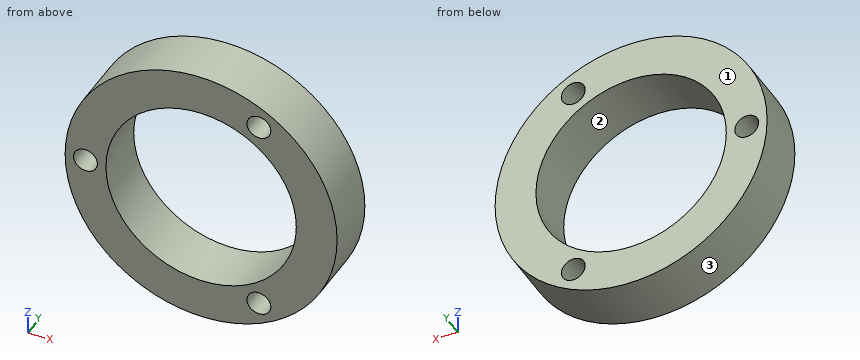
from build123d import *

# Parameters (mm, degrees)
SKETCH1_R           = 20
BOSS_EXTRUDE1_DEPTH = 8
SKETCH2_R           = 14
CUT_EXTRUDE1_DEPTH  = 8
CUT_EXTRUDE2_REACH  = 10
SKETCH3_R           = 1.75


with BuildPart() as part:
    # Sketch1 → Boss-Extrude1 (new body)
    with BuildSketch(Plane.XZ):
        with Locations((-34.143225555, 5.12970783)):
            Circle(SKETCH1_R)
    extrude(amount=BOSS_EXTRUDE1_DEPTH)

    # Sketch2 → Cut-Extrude1 (cut)
    with BuildSketch(Plane(origin=(0, 0, 0), x_dir=(1, 0, 0), z_dir=(0, 1, 0))):
        with Locations((-34.143225555, -5.12970783)):
            Circle(SKETCH2_R)
    extrude(amount=-CUT_EXTRUDE1_DEPTH, mode=Mode.SUBTRACT)

    # Sketch3 → Cut-Extrude2 (cut, up to next)
    with BuildSketch(Plane.XZ.offset(8), mode=Mode.PRIVATE) as cut_extrude2_sk1:
        with Locations((-25.643225555, 19.852139695)):
            Circle(SKETCH3_R)
    cut_extrude2_tool1 = extrude(cut_extrude2_sk1.sketch, amount=-CUT_EXTRUDE2_REACH, mode=Mode.PRIVATE) & part.part
    add(cut_extrude2_tool1.solids().sort_by_distance((-25.643226, -8, 19.85214))[0], mode=Mode.SUBTRACT)
    # Sketch3 → Cut-Extrude2 (cut, up to next)
    with BuildSketch(Plane.XZ.offset(8), mode=Mode.PRIVATE) as cut_extrude2_sk2:
        with Locations((-25.643225555, -9.592724034)):
            Circle(SKETCH3_R)
    cut_extrude2_tool2 = extrude(cut_extrude2_sk2.sketch, amount=-CUT_EXTRUDE2_REACH, mode=Mode.PRIVATE) & part.part
    add(cut_extrude2_tool2.solids().sort_by_distance((-25.643226, -8, -9.592724))[0], mode=Mode.SUBTRACT)
    # Sketch3 → Cut-Extrude2 (cut, up to next)
    with BuildSketch(Plane.XZ.offset(8), mode=Mode.PRIVATE) as cut_extrude2_sk3:
        with Locations((-51.143225555, 5.12970783)):
            Circle(SKETCH3_R)
    cut_extrude2_tool3 = extrude(cut_extrude2_sk3.sketch, amount=-CUT_EXTRUDE2_REACH, mode=Mode.PRIVATE) & part.part
    add(cut_extrude2_tool3.solids().sort_by_distance((-51.143226, -8, 5.129708))[0], mode=Mode.SUBTRACT)


solid = part.part
CAD build for the part. Positions are in the model's coordinates, mm. Face numbers are marked on the shaded views. Round coordinates to 2 decimals unless told otherwise and drop trailing zeros. Write each loop counter-clockwise with the first axis right and the second up, starting at its lowest first coordinate (ties: lowest second). Pieces come first, ordered by that corner, then holes. Notation, with made-up numbers: M -22,59.25 L -15,59.25 A22 ccw -15,91.25 Z; hole C 67.25,-16.5 d5. An arc over 180 degrees is marked long. Put each result on its own line as item: value. Start each with the question number.
1) Pin check, flat tips, straight feed: pin 1 Ø4 at (x, y) = (-43.5, -5) entering from +Z; pin 2 Ø4 at (x, y) = (-41, -7) entering from -Z; pin 3 Ø3 at (x, y) = (-37.5, -3.5) entering from +Z. Stop position of each tip, or through.
2) Saw through at A-A, the plane x = -44.5. Write the cut outline in (y, z).
3) Saw through at C-C, the plane y = -4. Write the cut outline in (x, z), and give its area (3 significant figures).
4) Saw through at D-D, the plane z = 23. Write the cut outline in (x, y).
5) Drill centre lines: probe 1 along Z at (x, y) = (-25.5, -4.5); probe 2 along Z at (x, y) = (-46, -5); probe 3 along Z at (x, y) = (-33.5, -5.25). Where is each one in solid material? Low to high. Write a range as [from, to].
6) Saw through at B-B, the plane z = 13. Write the cut outline in (x, y), and give its area (3 significant figures).
7) Pull direction Z, two halves, no side cores. Call the marked faces 1, 2 and 3: pulls with the +Z half, pulls with the -Z half, needs draft (parallel to the pull), parting line crosses it, or undercut.
Resolved:
1. pin 1: z = 23.73
1. pin 2: z = -14.27
1. pin 3: z = 25.04
2. outline: M -8,-11.98 L 0,-11.98 L 0,-4.29 L -8,-4.29 Z; M -8,14.55 L 0,14.55 L 0,22.24 L -8,22.24 Z
3. outline: C -34.14,5.13 d40; hole C -51.14,5.13 d3.5; hole C -34.14,5.13 d28; hole C -25.64,-9.59 d3.5; hole C -25.64,19.85 d3.5
3. area: 612 mm²
4. outline: M -43.12,-8 L -25.16,-8 L -25.16,0 L -43.12,0 Z
5. probe 1: [-12.91, -11.34], [-7.85, -5.88], [16.14, 18.11], [21.6, 23.17]
5. probe 2: [-10.98, -2.31], [12.57, 21.24]
5. probe 3: [-14.86, -8.86], [19.11, 25.12]
6. outline: M -52.53,-8 L -45.72,-8 L -45.72,0 L -52.53,0 Z; M -22.56,-8 L -15.76,-8 L -15.76,0 L -22.56,0 Z
6. area: 109 mm²
7. face 1: needs draft
7. face 2: undercut
7. face 3: parting line crosses it
